Answer from the drawing. Dimensions are ordinates in mm from the lowest x, y and z of the part. A direction names the side the tool comes from. Round coordinates to 2 decimals unless told otherwise and drop trailing zeros. Write each loop counter-clockwise with the first axis right and the second up, starting at its lowest first coordinate (ties: lowest second). Pieces come first, ordered by that corner, then holes. Notation, with made-up numbers: (-12, -8.75) -> (15, -8.75) arc R27 ccw to (15, 11.25) -> close; hole circle Ø2 at (53.25, 26). An arc over 180 degrees is marked (long way). Return JSON: item names as keys, results as strings. Group by question number.
(1) Straight lines are drawn through the part: line 1 (Y direction, x = 6.9, z = 10); line 2 (Z direction, x = 10, y = 9.75); line 3 (X direction, y = 13.5, z = 5.25). For each, find the intervals that lie inside material, in ascending order.
(2) A cutting plane is placed at A-A on z = 10. Give the vertices of the cut face in (x, y), then the cut area to 3 significant figures.
(3) For the marked faces 5, 6, 7 and 8, determine the directions among +Z, -Z, +X, -X, +Y, -Y from which every point of the face is accessible in a straight line to the end or side of a thin tool.
(4) Given pin 1 (2.5 mm diameter, centred on x = 11.5, y = 8, fed in from -Z); pin 2 (5 mm diameter, centred on y = 11, z = 10.5, fed in from +X); pin 3 (7 mm diameter, centred on y = 10.1, z = 10, fed in from -X); pin 4 (1.5 mm diameter, centred on x = 2.5, y = 5.5, fed in from -Z), each flat-ended and moving along its own axis, determine where each tip first touches the part or whether it passes through.
(5) A cutting plane is placed at C-C on y = 10.1. Give the vertices of the cut face in (x, z), then the cut area to 3 significant figures.
(6) The mould has two halves that part along Z. Classify the marked faces 1, 2, 3 and 4: released by +Z, released by -Z, zero draft, split by the parting line, or undercut.
(7) A cutting plane is placed at D-D on x = 9.5. Give the vertices of the cut face in (y, z).
(8) A cutting plane is placed at B-B on y = 15. Give the vertices of the cut face in (x, z).
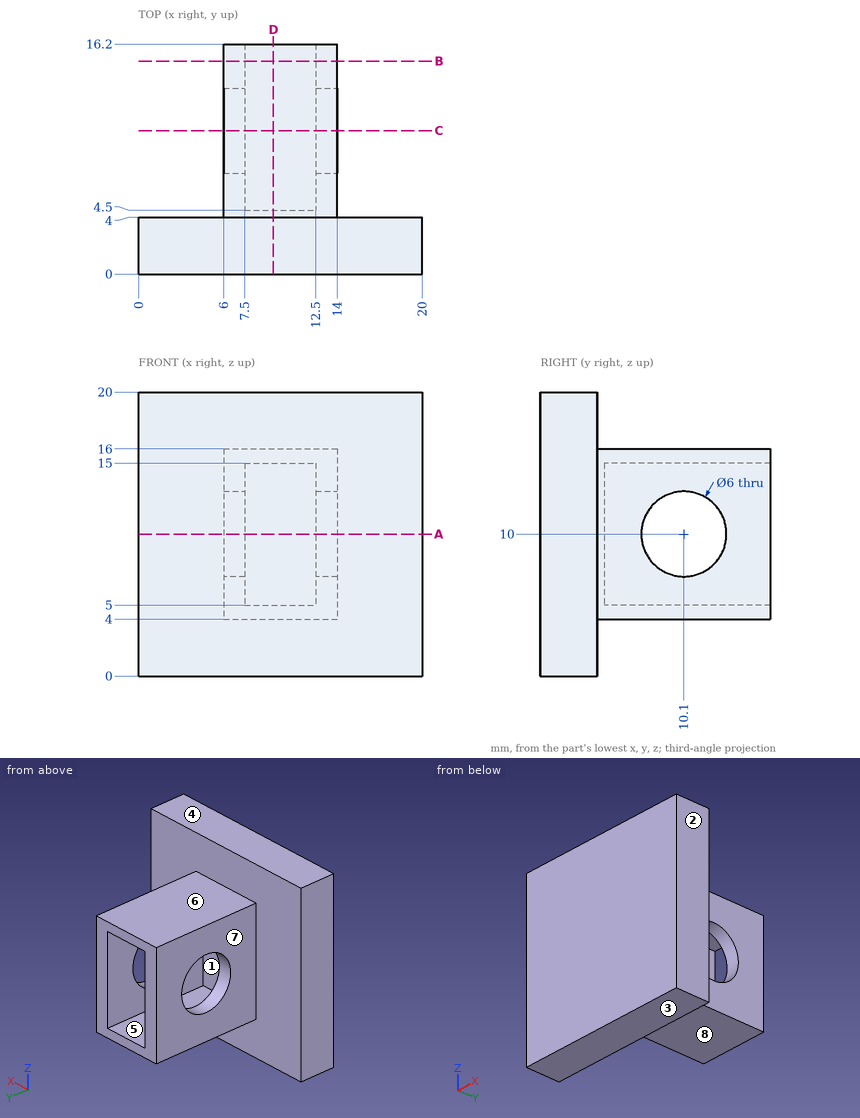
Checks:
{
 "1": {"line 1": "y = 0 to 7.1, 13.1 to 16.2", "line 2": "z = 4 to 5, 15 to 16", "line 3": "x = 6 to 7.5, 12.5 to 14"},
 "2": {"outline": "(0, 0) -> (20, 0) -> (20, 4) -> (14, 4) -> (14, 7.1) -> (12.5, 7.1) -> (12.5, 4.5) -> (7.5, 4.5) -> (7.5, 7.1) -> (6, 7.1) -> (6, 4) -> (0, 4) -> close; (6, 13.1) -> (7.5, 13.1) -> (7.5, 16.2) -> (6, 16.2) -> close; (12.5, 13.1) -> (14, 13.1) -> (14, 16.2) -> (12.5, 16.2) -> close", "area": "101 mm^2"},
 "3": {"face 5": "+Y", "face 6": "+Z, +X, -X, +Y", "face 7": "+Z, -Z, -X, +Y", "face 8": "-Z, +X, -X, +Y"},
 "4": {"pin 1": "stops at z = 4", "pin 2": "stops at x = 14", "pin 3": "stops at x = 6", "pin 4": "passes through"},
 "5": {"outline": "(6, 4) -> (14, 4) -> (14, 7) -> (12.5, 7) -> (12.5, 5) -> (7.5, 5) -> (7.5, 7) -> (6, 7) -> close; (6, 13) -> (7.5, 13) -> (7.5, 15) -> (12.5, 15) -> (12.5, 13) -> (14, 13) -> (14, 16) -> (6, 16) -> close", "area": "28.0 mm^2"},
 "6": {"face 1": "undercut", "face 2": "zero draft", "face 3": "released by -Z", "face 4": "released by +Z"},
 "7": {"outline": "(0, 0) -> (4, 0) -> (4, 4) -> (16.2, 4) -> (16.2, 5) -> (4.5, 5) -> (4.5, 15) -> (16.2, 15) -> (16.2, 16) -> (4, 16) -> (4, 20) -> (0, 20) -> close"},
 "8": {"outline": "(6, 4) -> (14, 4) -> (14, 16) -> (6, 16) -> close; hole (7.5, 5) -> (12.5, 5) -> (12.5, 15) -> (7.5, 15) -> close"}
}
